from build123d import *

# Parameters (mm, degrees)
BOSS_EXTRUDE1_DEPTH = 2


with BuildPart() as part:
    # Sketch1 → Boss-Extrude1 (new, symmetric)
    with BuildSketch(Plane.XY):
        with BuildLine():
            Line((-4, -3.7), (4, -3.7))
            ThreePointArc((4, -3.7), (7.7, 0), (4, 3.7))
            Line((4, 3.7), (-4, 3.7))
            ThreePointArc((-4, 3.7), (-7.7, 0), (-4, -3.7))
        make_face()
        with BuildLine():
            Line((-3.1, 2.224859546), (-3.1, 0.9))
            Line((-3.1, 0.9), (-1.775140454, 0.9))
            ThreePointArc((-1.775140454, 0.9), (-1.6, 0), (-1.775140454, -0.9))
            Line((-1.775140454, -0.9), (-3.1, -0.9))
            Line((-3.1, -0.9), (-3.1, -2.224859546))
            ThreePointArc((-3.1, -2.224859546), (-4, -2.4), (-4.9, -2.224859546))
            Line((-4.9, -2.224859546), (-4.9, -0.9))
            Line((-4.9, -0.9), (-6.224859546, -0.9))
            ThreePointArc((-6.224859546, -0.9), (-6.4, 0), (-6.224859546, 0.9))
            Line((-6.224859546, 0.9), (-4.9, 0.9))
            Line((-4.9, 0.9), (-4.9, 2.224859546))
            ThreePointArc((-4.9, 2.224859546), (-4, 2.4), (-3.1, 2.224859546))
        make_face(mode=Mode.SUBTRACT)
        with BuildLine():
            ThreePointArc((4.9, -2.224859546), (4, -2.4), (3.1, -2.224859546))
            Line((3.1, -2.224859546), (3.1, -0.9))
            Line((3.1, -0.9), (1.775140454, -0.9))
            ThreePointArc((1.775140454, -0.9), (1.6, 0), (1.775140454, 0.9))
            Line((1.775140454, 0.9), (3.1, 0.9))
            Line((3.1, 0.9), (3.1, 2.224859546))
            ThreePointArc((3.1, 2.224859546), (4, 2.4), (4.9, 2.224859546))
            Line((4.9, 2.224859546), (4.9, 0.9))
            Line((4.9, 0.9), (6.224859546, 0.9))
            ThreePointArc((6.224859546, 0.9), (6.4, 0), (6.224859546, -0.9))
            Line((6.224859546, -0.9), (4.9, -0.9))
            Line((4.9, -0.9), (4.9, -2.224859546))
        make_face(mode=Mode.SUBTRACT)
    extrude(amount=BOSS_EXTRUDE1_DEPTH, both=True)


solid = part.part
The listing builds one solid part. Answer for the finished solid, in the listing's coordinates (mm). A direction names the side the tool comes from. Coordinates: 2 decimals unless noted, no trailing zeros. Order: outer loops, then holes, each group sorted by start corner. A loop starts at its lowest first (then second) coordinate and runs counter-clockwise, first axis right, second up.
Q1. Given P1, Ø0.7, axis at x = -5.5, z = 0, coming from the -Y side; P2, Ø1.1, axis at y = 2, z = -1, coming from the +X side; P3, Ø1, axis at y = 0.5, z = -1.5, coming from the -X side; P4, Ø0.7, axis at y = 1.5, z = 0, coming from the -X side, each flat-ended and moving along its own axis, determine where each tip first touches the part or whether it passes through.
Q2. Which of the six approach directions +Z, -Z, +X, -X, +Y, -Y give full straight-line access (tool end or side, diameter ignored) to faces 1 (the face through (-7.7, 0.1, 0)), 2 (the face through (2, 0.9, 0))?
Q3. A cutting plane is placed at D-D, the plane y = 1.75. Write down the section's boundary in (x, z).
Q4. A cutting plane is placed at A-A, the plane y = 0. Write down the section's boundary in (x, z), and give its area (3 significant figures).
Q5. Consider line 1 (Y direction, x = 2.75, z = 1.5); line 2 (X direction, y = -0.75, z = -0.1); line 3 (X direction, y = -1.25, z = -1.2). Determine where each line is inside the solid, lowest interval first.
Q6. A cutting plane is placed at C-C, the plane z = -0.25. Write down the section's boundary in (x, y).
Q7. A cutting plane is placed at B-B, the plane x = -2.5. Write down the section's boundary in (y, z), and give its area (3 significant figures).
Q8. For a pull along Y with two mould halves and no side action, classify faces 3 (the face through (0, 3.7, 0)), 4 (the face through (-3.1, 2, 0)), 5 (the face through (0, 0, -2)), 6 (the face through (0, -3.7, 0)) as pulls with the +Y half, pulls with the -Y half, needs draft (parallel to the pull), parting line crosses it, or undercut.
Answers follow:
1. P1: stops at y = -3.52
1. P2: stops at x = 7.4
1. P3: stops at x = -7.7
1. P4: stops at x = -7.52
2. face 1: +Z, -Z, -X
2. face 2: +Z, -Z
3. outline: (-7.26, -2) - (-4.9, -2) - (-4.9, 2) - (-7.26, 2) - close; (-3.1, -2) - (3.1, -2) - (3.1, 2) - (-3.1, 2) - close; (4.9, -2) - (7.26, -2) - (7.26, 2) - (4.9, 2) - close
4. outline: (-7.7, -2) - (-6.4, -2) - (-6.4, 2) - (-7.7, 2) - close; (-1.6, -2) - (1.6, -2) - (1.6, 2) - (-1.6, 2) - close; (6.4, -2) - (7.7, -2) - (7.7, 2) - (6.4, 2) - close
4. area: 23.2 mm2
5. line 1: y = -3.7 to -0.9, 0.9 to 3.7
5. line 2: x = -7.62 to -6.28, -1.72 to 1.72, 6.28 to 7.62
5. line 3: x = -7.48 to -4.9, -3.1 to 3.1, 4.9 to 7.48
6. outline: (-4, -3.7) - (4, -3.7) arc R3.7 ccw to (4, 3.7) - (-4, 3.7) arc R3.7 ccw to start; hole (-6.22, -0.9) - (-4.9, -0.9) - (-4.9, -2.22) arc R2.4 ccw to (-3.1, -2.22) - (-3.1, -0.9) - (-1.78, -0.9) arc R2.4 ccw to (-1.78, 0.9) - (-3.1, 0.9) - (-3.1, 2.22) arc R2.4 ccw to (-4.9, 2.22) - (-4.9, 0.9) - (-6.22, 0.9) arc R2.4 ccw to start; hole (1.78, -0.9) - (3.1, -0.9) - (3.1, -2.22) arc R2.4 ccw to (4.9, -2.22) - (4.9, -0.9) - (6.22, -0.9) arc R2.4 ccw to (6.22, 0.9) - (4.9, 0.9) - (4.9, 2.22) arc R2.4 ccw to (3.1, 2.22) - (3.1, 0.9) - (1.78, 0.9) arc R2.4 ccw to start
7. outline: (-3.7, -2) - (-0.9, -2) - (-0.9, 2) - (-3.7, 2) - close; (0.9, -2) - (3.7, -2) - (3.7, 2) - (0.9, 2) - close
7. area: 22.4 mm2
8. face 3: pulls with the +Y half
8. face 4: undercut
8. face 5: needs draft
8. face 6: pulls with the -Y half
